```python
from build123d import *

# Parameters (mm, degrees)
F1_DEPTH = 25.4
F2_DEPTH = 25.4


with BuildPart() as f1:
    # F0 (on Top) → F1 (new body)
    with BuildSketch(Plane.XY):
        Polygon((20.612943, -13.130079), (22.096039, -10.443057), (23.230667, -7.591343), (23.998934, -4.619908), (24.388723, -1.575615), (24.393888, 1.493527), (24.014346, 4.539115), (23.256084, 7.513118), (22.131059, 10.368635), (20.657015, 13.060633), (18.857197, 15.546656), (16.759989, 17.7875), (14.398467, 19.747823), (11.809872, 21.396712), (9.035029, 22.708162), (6.117697, 23.661491), (3.103886, 24.241664), (0.041125, 24.439531), (-3.022285, 24.251973), (-6.038031, 23.681946), (-8.958554, 22.738441), (-11.737796, 21.436337), (-14.331925, 19.796169), (-16.700032, 17.843804), (-18.804768, 15.610031), (-20.612943, 13.130079), (-22.096039, 10.443057), (-23.230667, 7.591343), (-23.998934, 4.619908), (-24.388723, 1.575615), (-24.393888, -1.493527), (-24.014346, -4.539115), (-23.256084, -7.513118), (-22.131059, -10.368635), (-20.657015, -13.060633), (-18.857197, -15.546656), (-16.759989, -17.7875), (-14.398467, -19.747823), (-11.809872, -21.396712), (-9.035029, -22.708162), (-6.117697, -23.661491), (-3.103886, -24.241664), (-0.041125, -24.439531), (3.022285, -24.251973), (6.038031, -23.681946), (8.958554, -22.738441), (11.737796, -21.436337), (14.331925, -19.796169), (16.700032, -17.843804), (18.804768, -15.610031), align=None)
        Polygon((4.921291, 5.679472), (7.210608, 2.117225), (7.210608, -2.117225), (4.921291, -5.679472), (1.069499, -7.438527), (-3.121852, -6.835901), (-6.322036, -4.062926), (-7.515019, 0), (-6.322036, 4.062926), (-3.121852, 6.835901), (1.069499, 7.438527), align=None, mode=Mode.SUBTRACT)
    extrude(amount=F1_DEPTH)

    # F1_face (on face) → F2 (join)
    with BuildSketch(Plane.XY.offset(25.4)):
        Polygon((-23.998934, 4.619908), (-24.388723, 1.575615), (-24.393888, -1.493527), (-24.014346, -4.539115), (-23.256084, -7.513118), (-22.131059, -10.368635), (-20.657015, -13.060633), (-18.857197, -15.546656), (-16.759989, -17.7875), (-14.398467, -19.747823), (-11.809872, -21.396712), (-9.035029, -22.708162), (-6.117697, -23.661491), (-3.103886, -24.241664), (-0.041125, -24.439531), (3.022285, -24.251973), (6.038031, -23.681946), (8.958554, -22.738441), (11.737796, -21.436337), (14.331925, -19.796169), (16.700032, -17.843804), (18.804768, -15.610031), (20.612943, -13.130079), (22.096039, -10.443057), (23.230667, -7.591343), (23.998934, -4.619908), (24.388723, -1.575615), (24.393888, 1.493527), (24.014346, 4.539115), (23.256084, 7.513118), (22.131059, 10.368635), (20.657015, 13.060633), (18.857197, 15.546656), (16.759989, 17.7875), (14.398467, 19.747823), (11.809872, 21.396712), (9.035029, 22.708162), (6.117697, 23.661491), (3.103886, 24.241664), (0.041125, 24.439531), (-3.022285, 24.251973), (-6.038031, 23.681946), (-8.958554, 22.738441), (-11.737796, 21.436337), (-14.331925, 19.796169), (-16.700032, 17.843804), (-18.804768, 15.610031), (-20.612943, 13.130079), (-22.096039, 10.443057), (-23.230667, 7.591343), align=None)
        Polygon((1.069499, 7.438527), (4.921291, 5.679472), (7.210608, 2.117225), (7.210608, -2.117225), (4.921291, -5.679472), (1.069499, -7.438527), (-3.121852, -6.835901), (-6.322036, -4.062926), (-7.515019, 0), (-6.322036, 4.062926), (-3.121852, 6.835901), align=None, mode=Mode.SUBTRACT)
    extrude(amount=F2_DEPTH)


solid = f1.part
```
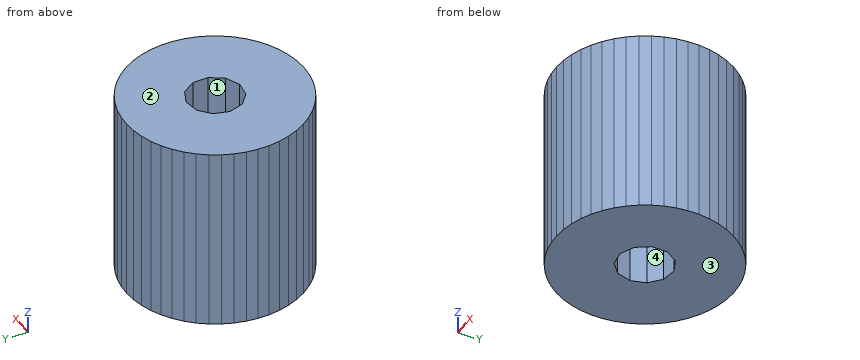
Work out the finished part from the listing and answer in its coordinate system (mm). Face numbers are marked on the shaded views. A direction names the side the tool comes from. Round coordinates to 2 decimals unless told otherwise and drop trailing zeros. Order: outer loops, then holes, each group sorted by start corner. A loop starts at its lowest first (then second) coordinate and runs counter-clockwise, first axis right, second up.
Q1. Find the intervals of material crossed by line 1 along Y through (x, z) = (-3, 32.5); line 2 along Y through (x, z) = (-5, 19.5); line 3 along X through (y, z) = (1, 36.5), in increasing order.
Solution:
line 1: y = -24.25 to -6.85, 6.85 to 24.25
line 2: y = -23.88 to -5.21, 5.21 to 23.88
line 3: x = -24.39 to -7.22, 7.21 to 24.39
Q2. A tool of negligible diameter and unlimited length cuts with its end or side. For the marked faces 1 and 2, from which of +Z, -Z, +X, -X, +Y, -Y can it reach the whole face along a straight path? Write none if from no direction.
Solution:
face 1: +Z, -Z
face 2: +Z, +X, -X, +Y, -Y
Q3. Given pin 1 Ø4 at (y, z) = (-14, 38) entering from +X; pin 2 Ø2 at (y, z) = (-14.5, 12) entering from +X; pin 3 Ø5 at (y, z) = (-13, 26.5) entering from +X; pin 4 Ø3.5 at (y, z) = (0.5, 13) entering from -X, each flat-ended and moving along its own axis, determine where each tip first touches the part or whether it passes through.
Solution:
pin 1: stops at x = 21.24
pin 2: stops at x = 20.34
pin 3: stops at x = 22.06
pin 4: stops at x = -24.39
Q4. The mould has two halves that part along X. Classify the marked faces 3 and 4: pulls with the +X half, pulls with the -X half, needs draft (parallel to the pull), parting line crosses it, or undercut.
Solution:
face 3: needs draft
face 4: undercut
Q5. A cutting plane is placed at B-B, the plane x = -10. Determine the outline of the cut face in (y, z).
Solution:
outline: (-22.25, 0) - (22.25, 0) - (22.25, 50.8) - (-22.25, 50.8) - close
Q6. A cutting plane is placed at A-A, the plane y = 11.5. Determine the outline of the cut face in (x, z), then the cut area to 3 significant figures.
Solution:
outline: (-21.51, 0) - (21.51, 0) - (21.51, 50.8) - (-21.51, 50.8) - close
area: 2,190 mm2
